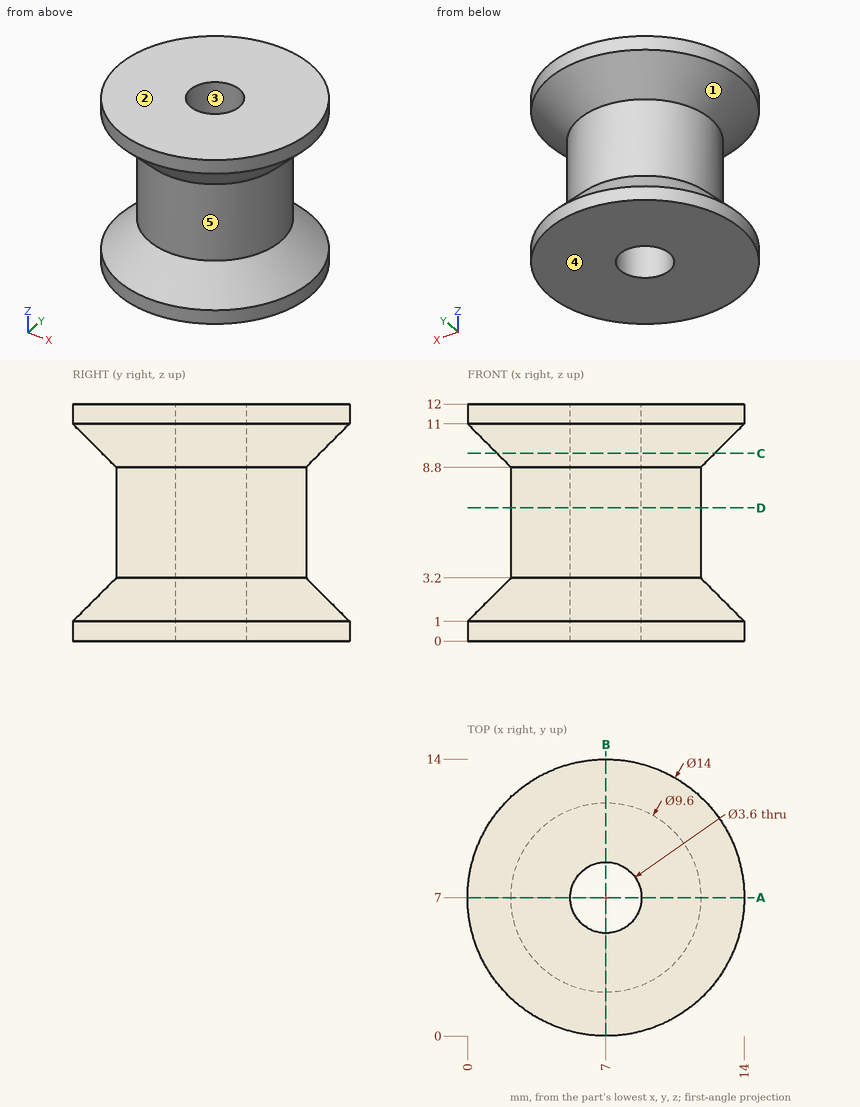
Geometry: see drawing. Coordinates: mm, zero at the bounding-box minimum. A direction names the side the tool comes from. Coordinates: 2 decimals unless noted, no trailing zeros. Loops run counter-clockwise (first coordinate to the right, second up) from the corner with the lowest first, then second, coordinate; pieces in that order, holes last. Notation, with made-up numbers: (45.25, -30.5) - (50.25, -30.5) arc R17 cw to (50.25, -14.5) - close; hole circle Ø5 at (-21, 8). An arc over 180 degrees is marked (long way). Return JSON: item names as keys, results as strings.
Q1. Material intervals for line 1 along Y through (x, z) = (7, 6.75); line 2 along Z through (x, y) = (1.75, 7); line 3 along X through (y, z) = (5.5, 6), sorted ascending.
Results:
{"line 1": "2.2 to 5.2, 8.8 to 11.8", "line 2": "0 to 2.75, 9.25 to 12", "line 3": "2.44 to 6.01, 7.99 to 11.56"}
Q2. Section D-D, the plane z = 6.75. Return loops of the section in (x, y).
Results:
{"outline": "circle Ø9.6 at (7, 7); hole circle Ø3.6 at (7, 7)"}
Q3. Contact query for flat-ended pins moving along their axis: P1, Ø2, axis at x = 11, z = 7, coming from the +Y side; P2, Ø3, axis at x = 3, y = 4, coming from the -Z side; P3, Ø2, axis at y = 2.5, z = 6, coming from the +X side; P4, Ø2, axis at x = 7, y = 7, coming from the -Z side. Output: stop coordinate, or through.
Results:
{"P1": "y = 10.75", "P2": "z = 0", "P3": "x = 10.28", "P4": "through"}
Q4. Section A-A, the plane y = 7. Return loops of the section in (x, z).
Results:
{"outline": "(0, 0) - (5.2, 0) - (5.2, 12) - (0, 12) - (0, 11) - (2.2, 8.8) - (2.2, 3.2) - (0, 1) - close; (8.8, 0) - (14, 0) - (14, 1) - (11.8, 3.2) - (11.8, 8.8) - (14, 11) - (14, 12) - (8.8, 12) - close"}
Q5. Access query for the marked faces 1 and 2. Directions: +Z, -Z, +X, -X, +Y, -Y. A direction counts if a zero-diameter tool reaches every point of the face in a straight line with its end or side. Return the directions, or none.
Results:
{"face 1": "none", "face 2": "+Z, +X, -X, +Y, -Y"}
Q6. Mould query, pull axis Z, two halves, no side actions, for the marked faces 3, 4 and 5. Classes: released by +Z, released by -Z, zero draft, split by the parting line, or undercut.
Results:
{"face 3": "zero draft", "face 4": "released by -Z", "face 5": "undercut"}
Q7. Section C-C, the plane z = 9.5. Return loops of the section in (x, y).
Results:
{"outline": "circle Ø11 at (7, 7); hole circle Ø3.6 at (7, 7)"}
